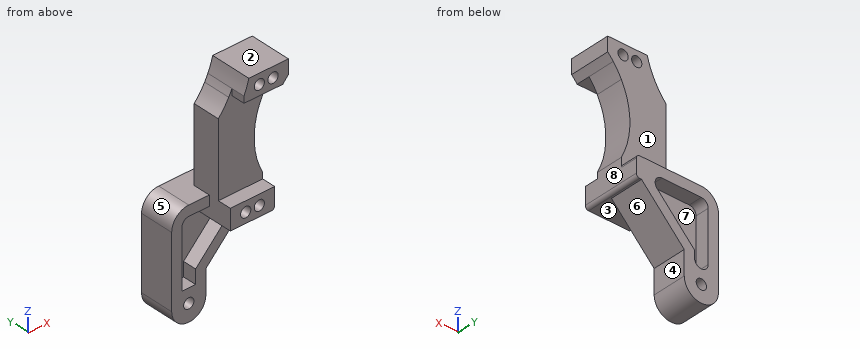
from build123d import *

# Parameters (mm, degrees)
SKETCH1_W             = 13
SKETCH1_H             = 6
SKETCH1_R             = 1.5
BOSS_EXTRUDE1_DEPTH   = 4
BOSS_EXTRUDE1_2_DEPTH = 4
BOSS_EXTRUDE2_START   = 4
SKETCH1_4_R           = 1.5
SKETCH1_4_W           = 13
SKETCH1_4_H           = 6
BOSS_EXTRUDE2_DEPTH   = 8
SKETCH2_R             = 1.5
BOSS_EXTRUDE3_DEPTH   = 5
BOSS_EXTRUDE4_START   = -5
SKETCH2_3_R           = 1.5
BOSS_EXTRUDE4_DEPTH   = 5
CUT_EXTRUDE1_DEPTH    = 4
FILLET1_R             = 1
FILLET2_R             = 1
FILLET3_R             = 2
BOSS_EXTRUDE5_START   = 11
SKETCH4_R             = 1.5
BOSS_EXTRUDE5_DEPTH   = 11


with BuildPart() as part:
    # Sketch1 → Boss-Extrude1 (new body)
    with BuildSketch(Plane(origin=(0, -9, 0), x_dir=(1, 0, 0), z_dir=(0, 1, 0))):
        with Locations((25.1, 41)):
            Rectangle(SKETCH1_W, SKETCH1_H)
        with Locations(Location((27.1, 41, 0), (0, 0, 270))):
            Circle(SKETCH1_R, mode=Mode.SUBTRACT)
        with Locations(Location((23.1, 41, 0), (0, 0, 270))):
            Circle(SKETCH1_R, mode=Mode.SUBTRACT)
    extrude(amount=BOSS_EXTRUDE1_DEPTH)



with BuildPart() as body_2:
    # Sketch1 → Boss-Extrude1 2 (new body)
    with BuildSketch(Plane(origin=(0, -9, 0), x_dir=(1, 0, 0), z_dir=(0, 1, 0))):
        with BuildLine():
            ThreePointArc((22.6, 10.089722494), (23.395394249, 8.075767946), (24.01171589, 6))
            Line((24.01171589, 6), (35.6, 6))
            Line((35.6, 6), (35.6, 10.18070798))
            ThreePointArc((35.6, 10.18070798), (34.768444056, 11.068532406), (33.986085046, 12))
            Line((33.986085046, 12), (31.6, 12))
            Line((31.6, 12), (22.6, 12))
            Line((22.6, 12), (22.6, 10.089722494))
        make_face()
        with Locations(Location((27.1, 9, 0), (0, 0, 270))):
            Circle(SKETCH1_R, mode=Mode.SUBTRACT)
        with Locations(Location((31.1, 9, 0), (0, 0, 270))):
            Circle(SKETCH1_R, mode=Mode.SUBTRACT)
    extrude(amount=BOSS_EXTRUDE1_2_DEPTH)


with BuildPart() as part_1:
    add(part.part)

    add(body_2.part)  # Boss-Extrude2 merges body 2
    # Sketch1<4> → Boss-Extrude2 (add)
    # profile 1 of 5: a face of its own
    with BuildSketch(Plane(origin=(0, -9, 0), x_dir=(1, 0, 0), z_dir=(0, 1, 0)).offset(BOSS_EXTRUDE2_START)):
        with BuildLine():
            ThreePointArc((22.6, 10.089722494), (23.395394249, 8.075767946), (24.01171589, 6))
            Line((24.01171589, 6), (35.6, 6))
            Line((35.6, 6), (35.6, 10.18070798))
            ThreePointArc((35.6, 10.18070798), (34.768444056, 11.068532406), (33.986085046, 12))
            Line((33.986085046, 12), (31.6, 12))
            Line((31.6, 12), (22.6, 12))
            Line((22.6, 12), (22.6, 10.089722494))
        make_face()
        with Locations(Location((27.1, 9, 0), (0, 0, 270))):
            Circle(SKETCH1_4_R, mode=Mode.SUBTRACT)
        with Locations(Location((31.1, 9, 0), (0, 0, 270))):
            Circle(SKETCH1_4_R, mode=Mode.SUBTRACT)
    # profile 2 of 5: a face of its own
    with BuildSketch(Plane(origin=(0, -9, 0), x_dir=(1, 0, 0), z_dir=(0, 1, 0)).offset(BOSS_EXTRUDE2_START)):
        with BuildLine():
            Line((21.646304534, 12), (22.6, 12))
            Line((22.6, 12), (31.6, 12))
            Line((31.6, 12), (31.6, 15.692235936))
            ThreePointArc((31.6, 15.692235936), (29.1, 26), (31.6, 36.307764064))
            Line((31.6, 36.307764064), (31.6, 38))
            Line((31.6, 38), (18.6, 38))
            Line((18.6, 38), (18.6, 16.327966805))
            ThreePointArc((18.6, 16.327966805), (20.239171953, 14.245645604), (21.646304534, 12))
        make_face()
    # profile 3 of 5: a face of its own
    with BuildSketch(Plane(origin=(0, -9, 0), x_dir=(1, 0, 0), z_dir=(0, 1, 0)).offset(BOSS_EXTRUDE2_START)):
        with BuildLine():
            Line((31.6, 15.692235936), (31.6, 12))
            Line((31.6, 12), (33.986085046, 12))
            ThreePointArc((33.986085046, 12), (32.702650951, 13.787702963), (31.6, 15.692235936))
        make_face()
    # profile 4 of 5: a face of its own
    with BuildSketch(Plane(origin=(0, -9, 0), x_dir=(1, 0, 0), z_dir=(0, 1, 0)).offset(BOSS_EXTRUDE2_START)):
        with BuildLine():
            ThreePointArc((21.646304534, 12), (22.143761114, 11.055150099), (22.6, 10.089722494))
            Line((22.6, 10.089722494), (22.6, 12))
            Line((22.6, 12), (21.646304534, 12))
        make_face()
    # profile 5 of 5: a face of its own
    with BuildSketch(Plane(origin=(0, -9, 0), x_dir=(1, 0, 0), z_dir=(0, 1, 0)).offset(BOSS_EXTRUDE2_START)):
        with Locations((25.1, 41)):
            Rectangle(SKETCH1_4_W, SKETCH1_4_H)
        with Locations(Location((27.1, 41, 0), (0, 0, 270))):
            Circle(SKETCH1_4_R, mode=Mode.SUBTRACT)
        with Locations(Location((23.1, 41, 0), (0, 0, 270))):
            Circle(SKETCH1_4_R, mode=Mode.SUBTRACT)
    extrude(amount=BOSS_EXTRUDE2_DEPTH)

    # Sketch2 → Boss-Extrude3 (add)
    with BuildSketch(Plane(origin=(0, 3, 0), x_dir=(1, 0, 0), z_dir=(0, 1, 0))):
        with BuildLine():
            Line((31.6, 38), (31.6, 44))
            Line((31.6, 44), (30.1, 44))
            Line((30.1, 44), (17.6, 57))
            Line((17.6, 57), (17.6, 64))
            ThreePointArc((17.6, 64), (12.6, 69), (7.6, 64))
            Line((7.6, 64), (7.6, 43))
            ThreePointArc((7.6, 43), (9.064466094, 39.464466094), (12.6, 38))
            Line((12.6, 38), (31.6, 38))
        make_face()
        with Locations(Location((12.6, 64, 0), (0, 0, 270))):
            Circle(SKETCH2_R, mode=Mode.SUBTRACT)
    extrude(amount=BOSS_EXTRUDE3_DEPTH)

    # Sketch2<3> → Boss-Extrude4 (add)
    with BuildSketch(Plane(origin=(0, 3, 0), x_dir=(1, 0, 0), z_dir=(0, 1, 0)).offset(BOSS_EXTRUDE4_START)):
        with BuildLine():
            Line((18.6, 38), (18.6, 44))
            Line((18.6, 44), (30.1, 44))
            Line((30.1, 44), (17.6, 57))
            Line((17.6, 57), (17.6, 64))
            ThreePointArc((17.6, 64), (12.6, 69), (7.6, 64))
            Line((7.6, 64), (7.6, 43))
            ThreePointArc((7.6, 43), (9.064466094, 39.464466094), (12.6, 38))
            Line((12.6, 38), (18.6, 38))
        make_face()
        with Locations(Location((12.6, 64, 0), (0, 0, 270))):
            Circle(SKETCH2_3_R, mode=Mode.SUBTRACT)
    extrude(amount=BOSS_EXTRUDE4_DEPTH)

    # Sketch3 → Cut-Extrude1 (cut)
    with BuildSketch(Plane(origin=(0, 8, 0), x_dir=(1, 0, 0), z_dir=(0, 1, 0))):
        with BuildLine():
            Line((10.6, 59.895837344), (14.6, 59.895837344))
            Line((14.6, 59.895837344), (14.6, 55.791674689))
            Line((14.6, 55.791674689), (28.822764124, 41))
            Line((28.822764124, 41), (12.6, 41))
            ThreePointArc((12.6, 41), (11.185786438, 41.585786438), (10.6, 43))
            Line((10.6, 43), (10.6, 59.895837344))
        make_face()
    cut_extrude1 = extrude(amount=-CUT_EXTRUDE1_DEPTH, mode=Mode.SUBTRACT)

    # Fillet1
    fillet1_edges = [part_1.edges().sort_by_distance(p)[0] for p in [
        (31.6, -0.5, -44),
    ]]
    fillet(fillet1_edges, radius=FILLET1_R)

    # Fillet2
    fillet2_edges = [part_1.edges().sort_by_distance(p)[0] for p in [
        (31.6, 5.5, -38),
    ]]
    fillet(fillet2_edges, radius=FILLET2_R)

    # Fillet3
    fillet3_edges = [part_1.edges().sort_by_distance(p)[0] for p in [
        (14.6, 6, -59.895837344),
        (10.6, 6, -59.895837344),
        (28.822764124, 6, -41),
    ]]
    fillet(fillet3_edges, radius=FILLET3_R - 0.0001)  # a hair under: the kernel refuses the full size

    # Mirror2: Cut-Extrude1 across plane
    add(cut_extrude1.mirror(Plane.ZX.offset(3)), mode=Mode.SUBTRACT)

    # Sketch4 → Boss-Extrude5 (add)
    with BuildSketch(Plane.XZ.offset(-2).offset(BOSS_EXTRUDE5_START)):
        with BuildLine():
            Line((18.6, -44), (30.6, -44))
            ThreePointArc((30.6, -44), (31.307106781, -43.707106781), (31.6, -43))
            Line((31.6, -43), (31.6, -38))
            Line((31.6, -38), (18.6, -38))
            Line((18.6, -38), (18.6, -44))
        make_face()
        with Locations(Location((23.1, -41, 0), (0, 0, 90))):
            Circle(SKETCH4_R, mode=Mode.SUBTRACT)
        with Locations(Location((27.1, -41, 0), (0, 0, 90))):
            Circle(SKETCH4_R, mode=Mode.SUBTRACT)
    extrude(amount=-BOSS_EXTRUDE5_DEPTH)


solid = part_1.part
Geometry: final body of the model. Coordinates: model frame, mm. Face numbers are marked on the shaded views. A direction names the side the tool comes from. Round coordinates to 2 decimals unless told otherwise and drop trailing zeros. Loops run counter-clockwise (first coordinate to the right, second up) from the corner with the lowest first, then second, coordinate; pieces in that order, holes last. Notation, with made-up numbers: M -33.5,54.25 L -9.5,54.25 A25 cw -9.5,81.25 Z; hole C 85.25,19 d7. An arc over 180 degrees is marked long. Put each result on its own line as item: value. Start each with the question number.
(1) Draft query along Z for the marked faces 6, 7 and 8. Return one class per face: +Z half, -Z half, draft (parallel to the pull), parting line (faces both ways), or undercut.
(2) Contact query for flat-ended pins moving along their axis: pin 1 Ø9.5 at (y, z) = (-2.5, -28.5) entering from -X; pin 2 Ø4.5 at (y, z) = (6.5, -51) entering from +X; pin 3 Ø2.5 at (x, z) = (31.1, -9) entering from -Y; pin 4 Ø1.5 at (y, z) = (-1, -20.5) entering from +X. Output: stop coordinate, or through.
(3) Section query A-A (y = -6.25). Return loops of the section in (x, z), then the cut area to 3 significant figures.
(4) Set-up query: the marked faces 1, 2, 3, 4 and 5. Return all of +Z, -Z, +X, -X, +Y, -Y with unobstructed straight access to the full face (end or side cutting, diameter ignored); none if empty.
(5) Section query B-B (x = 27.1). Return loops of the section in (y, z), then the cut area to 3 significant figures.
(6) Material intervals for line 1 along Z through (x, y) = (31.5, 1); line 2 along Z through (x, y) = (13.5, 0.25); line 3 along X through (y, z) = (-6, -9), sorted ascending. Write a range as [from, to].
(7) Section query C-C (y = 5.75). State how many separate pieces and enclosed holes the cut face has, then the cut area to 3 significant figures.
(8) Section query D-D (y = 1.25). Return loops of the section in (x, z), then the cut area to 3 significant figures.
Findings below:
1. face 6: -Z half
1. face 7: undercut
1. face 8: draft
2. pin 1: stops at x = 18.6
2. pin 2: stops at x = 25.53
2. pin 3: passes through
2. pin 4: stops at x = 29.99
3. outline: M 18.6,-44 L 30.6,-44 A1 ccw 31.6,-43 L 31.6,-38 L 18.6,-38 Z; M 22.6,-12 L 33.99,-12 A22.5 cw 35.6,-10.18 L 35.6,-6 L 24.01,-6 A24.75 cw 22.6,-10.09 Z; hole C 23.1,-41 d3; hole C 27.1,-41 d3; hole C 27.1,-9 d3; hole C 31.1,-9 d3
3. area: 123 mm2
4. face 1: +Z, +X, -X, +Y
4. face 2: +Z, +X, -X, +Y, -Y
4. face 3: -Y
4. face 4: -Z, +X, +Y, -Y
4. face 5: +Z, -X, +Y, -Y
5. outline: M -9,-44 L -2,-44 L -2,-47.12 L 8,-47.12 L 8,-38 L 3,-38 L 3,-10.5 L -9,-10.5 L -9,-12 L -5,-12 L -5,-38 L -9,-38 L -9,-39.5 L 3,-39.5 L 3,-42.5 L -9,-42.5 Z; M -9,-7.5 L 3,-7.5 L 3,-6 L -9,-6 Z
5. area: 341 mm2
6. line 1: z = [-43.44, -36.11], [-15.89, -10.45], [-7.55, -6]
6. line 2: z = [-68.92, -65.2], [-62.8, -59.9], [-41, -38]
6. line 3: x = [23.06, 25.6], [28.6, 29.6], [32.6, 35.6]
7. separate pieces: 1
7. enclosed holes: 2
7. area: 278 mm2
8. outline: M 7.6,-64 A5 ccw 17.6,-64 L 17.6,-57 L 30.1,-44 L 30.6,-44 A1 ccw 31.6,-43 L 31.6,-36.31 A22.5 cw 35.6,-10.18 L 35.6,-6 L 24.01,-6 A24.75 cw 18.6,-16.33 L 18.6,-38 L 12.6,-38 A5 ccw 7.6,-43 Z; hole M 10.6,-59.9 L 14.6,-59.9 L 14.6,-55.79 L 25.94,-44 L 18.6,-44 L 18.6,-41 L 12.6,-41 A2 ccw 10.6,-43 Z; hole C 12.6,-64 d3; hole C 23.1,-41 d3; hole C 27.1,-41 d3; hole C 27.1,-9 d3; hole C 31.1,-9 d3
8. area: 644 mm2
